Drawing for the job (mm, zero at the part's lowest x, y, z). A direction names the side the tool comes from. Coordinates: 2 decimals unless noted, no trailing zeros. Loops run counter-clockwise (first coordinate to the right, second up) from the corner with the lowest first, then second, coordinate; pieces in that order, holes last. Notation, with made-up numbers: (-14, -8.5) -> (4, -8.5) arc R18 cw to (4, 18.5) -> close; hole circle Ø5 at (-28, -11). An arc over 180 degrees is marked (long way). Write item = value, one per line. Start each with the question number.
(1) Drill centre lines: line 1 (X direction, y = 3, z = 4.5); line 2 (X direction, y = 4.5, z = 7); line 3 (Z direction, x = 2.75, y = 3). Where is each one in solid material? Low to high. Write a range as from..to.
(2) Flat gauge pins, fed straight in: P1, Ø1.2, axis at x = 2.5, y = 5, coming from the -Z side; P2, Ø3, axis at x = 15, z = 7, coming from the -Y side; P3, Ø0.6, axis at x = 9, y = 6, coming from the -Z side. Where does each tip first touch, or does it go through?
(3) Band-saw the part on A-A (x = 7). Write the cut outline in (y, z).
(4) Band-saw the part on C-C (z = 7.25). Write the cut outline in (x, y), and give its area (3 significant figures).
(5) Tool access for the marked faces 5, 6 and 7: list every direction of +Z, -Z, +X, -X, +Y, -Y with a clear straight run to the whole face (end or side of a thin tool).
(6) Band-saw the part on B-B (y = 4). Write the cut outline in (x, z).
(7) Pull direction X, two halves, no side cores. Call the marked faces 1, 2, 3 and 4: +X half, -X half, draft (parallel to the pull), parting line (faces both ways), or undercut.
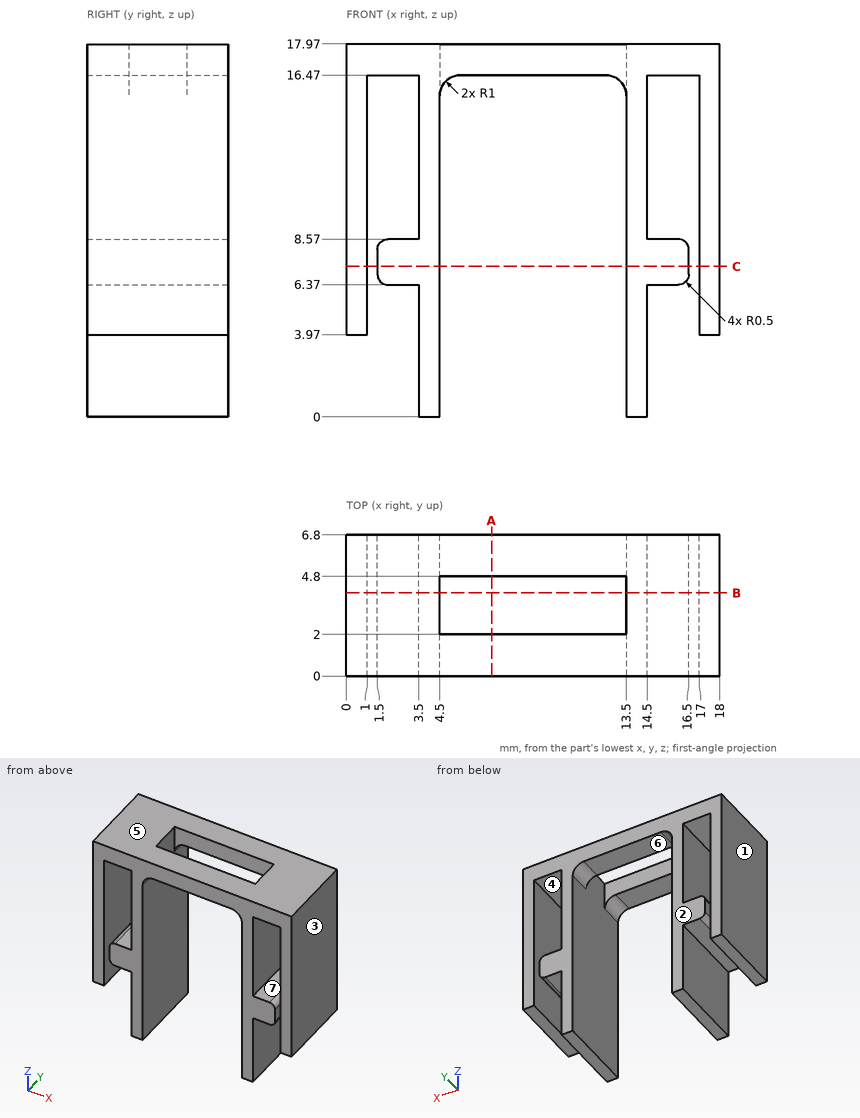
Findings below:
q1.line_1 = 0..1, 3.5..4.5, 13.5..14.5, 17..18
q1.line_2 = 0..1, 1.5..4.5, 13.5..16.5, 17..18
q1.line_3 = 6.37..8.57, 16.47..17.97
q2.P1 = 6.37
q2.P2 = 0
q2.P3 = 16.47
q3.outline = (0, 16.47) -> (2, 16.47) -> (2, 17.97) -> (0, 17.97) -> close; (4.8, 16.47) -> (6.8, 16.47) -> (6.8, 17.97) -> (4.8, 17.97) -> close
q4.outline = (0, 0) -> (1, 0) -> (1, 6.8) -> (0, 6.8) -> close; (1.5, 0) -> (4.5, 0) -> (4.5, 6.8) -> (1.5, 6.8) -> close; (13.5, 0) -> (16.5, 0) -> (16.5, 6.8) -> (13.5, 6.8) -> close; (17, 0) -> (18, 0) -> (18, 6.8) -> (17, 6.8) -> close
q4.area = 54.4 mm²
q5.face_5 = +Z, +X, -X, +Y, -Y
q5.face_6 = -Z, +Y, -Y
q5.face_7 = +Y, -Y
q6.outline = (0, 3.97) -> (1, 3.97) -> (1, 16.47) -> (3.5, 16.47) -> (3.5, 8.57) -> (2, 8.57) arc R0.5 ccw to (1.5, 8.07) -> (1.5, 6.87) arc R0.5 ccw to (2, 6.37) -> (3.5, 6.37) -> (3.5, 0) -> (4.5, 0) -> (4.5, 17.97) -> (0, 17.97) -> close; (13.5, 0) -> (14.5, 0) -> (14.5, 6.37) -> (16, 6.37) arc R0.5 ccw to (16.5, 6.87) -> (16.5, 8.07) arc R0.5 ccw to (16, 8.57) -> (14.5, 8.57) -> (14.5, 16.47) -> (17, 16.47) -> (17, 3.97) -> (18, 3.97) -> (18, 17.97) -> (13.5, 17.97) -> close
q7.face_1 = -X half
q7.face_2 = draft
q7.face_3 = +X half
q7.face_4 = undercut
